Work out the finished part from the listing and answer in its coordinate system (mm). A direction names the side the tool comes from. Round coordinates to 2 decimals unless told otherwise and drop trailing zeros. Write each loop counter-clockwise with the first axis right and the second up, starting at its lowest first coordinate (ties: lowest second). Pieces come first, ordered by that corner, then holes. Notation, with made-up numbers: (43, 15.25) -> (89, 15.25) arc R17 ccw to (89, 27.25) -> close; hole circle Ø10 at (-5, 57.25). An arc over 180 degrees is marked (long way). One line per item, written item: value.
```python
from build123d import *

# Parameters (mm, degrees)
SKETCH_1_W          = 78
SKETCH_1_H          = 55
EXTRUDE_1_DEPTH     = 22
SKETCH_2_W          = 74
SKETCH_2_H          = 51
CUT_EXTRUDE_1_DEPTH = 20
SKETCH_4_R          = 4
CUT_EXTRUDE_2_DEPTH = 20
SKETCH_5_R          = 2
CUT_EXTRUDE_4_DEPTH = 23


with BuildPart() as part:
    # 草图1 → 凸台-拉伸1 (new body)
    with BuildSketch(Plane(origin=(0, 0, 0), x_dir=(1, 0, 0), z_dir=(0, 1, 0))):
        with Locations((39, 27.5)):
            Rectangle(SKETCH_1_W, SKETCH_1_H)
    extrude(amount=EXTRUDE_1_DEPTH)

    # 草图2 → 切除-拉伸1 (cut)
    with BuildSketch(Plane(origin=(0, 22, 0), x_dir=(1, 0, 0), z_dir=(0, 1, 0))):
        with Locations((39, 27.5)):
            Rectangle(SKETCH_2_W, SKETCH_2_H)
    extrude(amount=-CUT_EXTRUDE_1_DEPTH, mode=Mode.SUBTRACT)

    # 草图4 → 切除-拉伸2 (cut)
    with BuildSketch(Plane(origin=(0, 22, 0), x_dir=(1, 0, 0), z_dir=(0, 1, 0))):
        with Locations((5, 9)):
            Circle(SKETCH_4_R)
        with Locations((5, 46)):
            Circle(SKETCH_4_R)
        with Locations((73, 46)):
            Circle(SKETCH_4_R)
        with Locations((73, 9)):
            Circle(SKETCH_4_R)
    extrude(amount=-CUT_EXTRUDE_2_DEPTH, mode=Mode.SUBTRACT)

    # 草图5 → 切除-拉伸4 (cut, through all)
    with BuildSketch(Plane(origin=(0, 22, 0), x_dir=(1, 0, 0), z_dir=(0, 1, 0))):
        with Locations((5, 9)):
            Circle(SKETCH_5_R)
        with Locations((5, 46)):
            Circle(SKETCH_5_R)
        with Locations((73, 46)):
            Circle(SKETCH_5_R)
        with Locations((73, 9)):
            Circle(SKETCH_5_R)
    extrude(amount=-CUT_EXTRUDE_4_DEPTH, mode=Mode.SUBTRACT)


solid = part.part
```
(1) Find section D-D on x = 20. Give the vertices of the cut face in (y, z).
Reported:
outline: (0, -55) -> (22, -55) -> (22, -53) -> (2, -53) -> (2, -2) -> (22, -2) -> (22, 0) -> (0, 0) -> close
(2) A flat-ended cylindrical pin translates along its axis: pin 1 Ø4.5 at (x, z) = (5, -9) entering from +Y. Find the tip coordinate at first contact, or state that the pin passes through.
Reported:
pin 1: stops at y = 2
(3) Consider probe 1 along Z at (x, y) = (73, 0.65); probe 2 along X at (y, z) = (0.6, -9); probe 3 along Z at (x, y) = (45, 14.25). Determine where each line is inside the solid, lowest interval first.
Reported:
probe 1: z = -55 to -48, -44 to -11, -7 to 0
probe 2: x = 0 to 3, 7 to 71, 75 to 78
probe 3: z = -55 to -53, -2 to 0
(4) A tool of negligible diameter and unlimited length cuts with its end or side. For faces 4 (the face through (5, 1, -44)), 5 (the face through (77, 12, -46)), from which of +Z, -Z, +X, -X, +Y, -Y can it reach the whole face along a straight path? Write none if from no direction.
Reported:
face 4: +Y, -Y
face 5: +Y
(5) Find section A-A on z = -9. Give the vertices of the cut face in (x, y), plus the area to 3 significant figures.
Reported:
outline: (0, 0) -> (3, 0) -> (3, 2) -> (1, 2) -> (1, 22) -> (0, 22) -> close; (7, 0) -> (71, 0) -> (71, 2) -> (7, 2) -> close; (75, 0) -> (78, 0) -> (78, 22) -> (77, 22) -> (77, 2) -> (75, 2) -> close
area: 180 mm2
(6) For a pull along X with two mould halves and no side action, classify faces 1 (the face through (38, 11, 0)), 2 (the face through (77, 12, -9)), 3 (the face through (78, 11, -27)) as pulls with the +X half, pulls with the -X half, needs draft (parallel to the pull), parting line crosses it, or undercut.
Reported:
face 1: needs draft
face 2: undercut
face 3: pulls with the +X half
(7) Find section C-C on y = 5.5. Give the vertices of the cut face in (x, z).
Reported:
outline: (0, -55) -> (78, -55) -> (78, 0) -> (0, 0) -> close; hole (2, -53) -> (76, -53) -> (76, -48.65) arc R4 ccw to (76, -43.35) -> (76, -11.65) arc R4 ccw to (76, -6.35) -> (76, -2) -> (2, -2) -> (2, -6.35) arc R4 ccw to (2, -11.65) -> (2, -43.35) arc R4 ccw to (2, -48.65) -> close
(8) Find section B-B on x = 5. Give the vertices of the cut face in (y, z).
Reported:
outline: (0, -55) -> (22, -55) -> (22, -53) -> (2, -53) -> (2, -48) -> (0, -48) -> close; (0, -44) -> (2, -44) -> (2, -11) -> (0, -11) -> close; (0, -7) -> (2, -7) -> (2, -2) -> (22, -2) -> (22, 0) -> (0, 0) -> close
